The listing builds one solid part. Answer for the finished solid, in the listing's coordinates (mm). A direction names the side the tool comes from. Round coordinates to 2 decimals unless told otherwise and drop trailing zeros. Loops run counter-clockwise (first coordinate to the right, second up) from the corner with the lowest first, then second, coordinate; pieces in that order, holes last. Notation, with made-up numbers: M -17.5,52 L -6.5,52 A22 cw -6.5,64 Z; hole C 6.5,8.25 d10. An arc over 180 degrees is marked long. Put each result on its own line as item: value. Start each with the question number.
(1) Which of the six approach directions +Z, -Z, +X, -X, +Y, -Y give full straight-line access (tool end or side, diameter ignored) to faces 4 (the face through (10, -2, 0)), 5 (the face through (-12, -2, 5.08)), 6 (the face through (19.05, -2, -1)), 7 (the face through (7.575, -1.565, 8.539)), 8 (the face through (0, -2, 12.192))?
(2) Straight lines are drawn through the part: line 1 (X direction, y = -0.35, z = -4) (3 decimals); line 2 (X direction, y = -2.3, z = -2); line 3 (Z direction, x = 3, y = -0.4). For each, find the intervals that lie inside material, in ascending order.
(3) Flat-ended cylindrical pins translate along their axes: P1, Ø0.6, axis at x = -12, y = -2, coming from the +Z side; P2, Ø0.6, axis at y = -1, z = 12.5, coming from the -X side; P3, Ø1.6, axis at x = -6.5, y = -1, coming from the +Z side. Find the tip coordinate at first contact, or state that the pin passes through.
(4) Section C-C, the plane y = -2.15 is taken. Count the separate pieces of the cut face and the enclosed holes in it, then the cut area to 3 significant figures.
(5) Determine the mould class of faces 1 (the face through (-17.14, -1.57, 3.27)), 2 (the face through (5.715, -2, -4)), 3 (the face through (0, -3.175, 4)) for opening direction X: released by +X, released by -X, zero draft, split by the parting line, or undercut.
(6) Section D-D, the plane z = 8 is taken. Determine the outline of the cut face in (x, y) (3 decimals).
(7) Section B-B, the plane z = -3.75 is taken. Determine the outline of the cut face in (x, y) (3 decimals), then the cut area to 3 significant figures.
(8) Section A-A, the plane x = -4 is taken. Determine the outline of the cut face in (y, z) (3 decimals), then the cut area to 3 significant figures.
```python
from build123d import *

# Parameters (mm, degrees)
F1_DEPTH = 3.175


with BuildPart() as f1:
    # F0 (on Front) → F1 (new body)
    with BuildSketch(Plane.XZ):
        with BuildLine():
            ThreePointArc((19.05, 3.81), (18.6780256121, 4.7080256121), (17.78, 5.08))
            Line((17.78, 5.08), (11.43, 5.08))
            Line((11.43, 5.08), (-11.43, 5.08))
            Line((-11.43, 5.08), (-12.7, 5.08))
            ThreePointArc((-12.7, 5.08), (-17.1901280605, 3.2201280605), (-19.05, -1.27))
            Line((-19.05, -1.27), (-19.05, -5.08))
            Line((-19.05, -5.08), (-13.335, -5.08))
            Line((-13.335, -5.08), (-13.335, -3.048))
            ThreePointArc((-13.335, -3.048), (-12.4422614691, -0.8927385309), (-10.287, 0))
            Line((-10.287, 0), (-8.763, 0))
            ThreePointArc((-8.763, 0), (-6.6077385309, -0.8927385309), (-5.715, -3.048))
            Line((-5.715, -3.048), (-5.715, -5.08))
            Line((-5.715, -5.08), (5.715, -5.08))
            Line((5.715, -5.08), (5.715, -3.048))
            ThreePointArc((5.715, -3.048), (6.6077385309, -0.8927385309), (8.763, 0))
            Line((8.763, 0), (10.287, 0))
            ThreePointArc((10.287, 0), (12.4422614691, -0.8927385309), (13.335, -3.048))
            Line((13.335, -3.048), (13.335, -5.08))
            Line((13.335, -5.08), (19.05, -5.08))
            Line((19.05, -5.08), (19.05, 3.81))
        make_face()
        Polygon((-11.43, 5.08), (11.43, 5.08), (7.8767356449, 12.7), (7.62, 12.7), (7.62, 12.192), (0, 12.192), (-7.62, 12.192), (-7.62, 12.7), (-7.8767356449, 12.7), align=None)
        Polygon((-1.016, 6.35), (-8.5957253428, 6.35), (-6.5822088749, 10.668), (-1.016, 10.668), align=None, mode=Mode.SUBTRACT)
        Polygon((8.5957253428, 6.35), (1.016, 6.35), (1.016, 10.668), (6.5822088749, 10.668), align=None, mode=Mode.SUBTRACT)
    extrude(amount=F1_DEPTH)


solid = f1.part
```
Recorded:
1. face 4: -Z, +Y, -Y
1. face 5: +Z, -X, +Y, -Y
1. face 6: +Z, -Z, +X, +Y, -Y
1. face 7: +Y, -Y
1. face 8: +Z, +Y, -Y
2. line 1: x = -19.05 to -13.335, -5.715 to 5.715, 13.335 to 19.05
2. line 2: x = -19.05 to -13.15, -5.9 to 5.9, 13.15 to 19.05
2. line 3: z = -5.08 to 6.35, 10.67 to 12.19
3. P1: stops at z = 5.08
3. P2: stops at x = -8.11
3. P3: stops at z = 12.19
4. separate pieces: 1
4. enclosed holes: 2
4. area: 391 mm²
5. face 1: released by -X
5. face 2: undercut
5. face 3: zero draft
6. outline: M -10.068,-3.175 L -7.826,-3.175 L -7.826,0 L -10.068,0 Z; M -1.016,-3.175 L 1.016,-3.175 L 1.016,0 L -1.016,0 Z; M 7.826,-3.175 L 10.068,-3.175 L 10.068,0 L 7.826,0 Z
7. outline: M -19.05,-3.175 L -13.335,-3.175 L -13.335,0 L -19.05,0 Z; M -5.715,-3.175 L 5.715,-3.175 L 5.715,0 L -5.715,0 Z; M 13.335,-3.175 L 19.05,-3.175 L 19.05,0 L 13.335,0 Z
7. area: 72.6 mm²
8. outline: M -3.175,-5.08 L 0,-5.08 L 0,6.35 L -3.175,6.35 Z; M -3.175,10.668 L 0,10.668 L 0,12.192 L -3.175,12.192 Z
8. area: 41.1 mm²
